```python
from build123d import *

# Parameters (mm, degrees)
F0_W     = 53.4262955189
F0_H     = 38.6142134666
F1_DEPTH = 37.0909944177
F2_R     = 12.7
F3_T     = -2.54


# Not quite as in the source:
# - a shell that OpenCascade refuses in one call is made with other operations: the cavity is built on its own and cut out


with BuildPart() as f1:
    # F0 (on Top) → F1 (new body)
    with BuildSketch(Plane.XY):
        with Locations((-26.7131477594, 19.3071067333)):
            Rectangle(F0_W, F0_H)
    extrude(amount=F1_DEPTH)

    # F2
    f2_edges = [f1.edges().sort_by_distance(p)[0] for p in [
        (-53.426296, 38.614213, 18.545497),
        (-53.426296, 0, 18.545497),
        (-53.426296, 19.307107, 0),
        (-53.426296, 19.307107, 37.090994),
    ]]
    fillet(f2_edges, radius=F2_R)

    # F3: a shell. OpenCascade refuses it in one call, so the cavity is built on its own and cut out:
    # the body offset inwards by the wall thickness, plus a prism from it out through each open face.
    f3_core = offset(f1.part, amount=F3_T, mode=Mode.PRIVATE)
    f3_exits = [f3_core.faces().sort_by_distance(p)[0] for p in [
        (-21.633148, 19.307107, 34.550994),
    ]]
    add(f3_core, mode=Mode.SUBTRACT)
    extrude(f3_exits, amount=-F3_T, mode=Mode.SUBTRACT)


solid = f1.part
```
Input: part model. Units: mm. Frame: model coordinates. A direction names the side the tool comes from. Give positions to 0.01 mm unless a question says otherwise; leave off trailing zeros. Order: outer loops, then holes, each group sorted by start corner. A loop starts at its lowest first (then second) coordinate and runs counter-clockwise, first axis right, second up. Notation, with made-up numbers: M 86.25,77.5 L 122.25,77.5 A28 cw 122.25,112.5 Z; hole C 18,38.25 d8. An arc over 180 degrees is marked long. Return JSON: item names as keys, results as strings.
1) Mould query, pull axis X, two halves, no side actions, for faces 4 (the face through (-48.125, 2.377, 18.805)), 5 (the face through (-21, 20, 0)), 6 (the face through (-46.645, 34.172, 18.77)). Classes: released by +X, released by -X, zero draft, split by the parting line, or undercut.
Taken from the geometry:
{"face 4": "released by -X", "face 5": "zero draft", "face 6": "undercut"}
2) Section query A-A on z = 19. Output: boundary loops of the cut face in (x, y).
Taken from the geometry:
{"outline": "M -53.43,12.7 A12.7 ccw -40.73,0 L 0,0 L 0,38.61 L -40.73,38.61 A12.7 ccw -53.43,25.91 Z; hole M -50.89,12.7 A10.16 ccw -40.73,2.54 L -2.54,2.54 L -2.54,36.07 L -40.73,36.07 A10.16 ccw -50.89,25.91 Z"}
3) Section query D-D on x = -42.5. Output: boundary loops of the cut face in (y, z).
Taken from the geometry:
{"outline": "M 0.12,0.12 L 38.49,0.12 L 38.49,36.97 L 0.12,36.97 Z; hole M 2.7,2.7 L 35.92,2.7 L 35.92,34.39 L 2.7,34.39 Z"}
4) Access query for faces 1 (the face through (-46.64, 19.54, 4.44)), 2 (the face through (-40.726, 19, 36)), 3 (the face through (-2, 17, 37.091)). Directions: +Z, -Z, +X, -X, +Y, -Y. A direction counts if a zero-diameter tool reaches every point of the face in a straight line with its end or side. Return the directions, or none.
Taken from the geometry:
{"face 1": "none", "face 2": "+Z", "face 3": "+Z, +X, -X, +Y, -Y"}
5) Contact query for flat-ended pins moving along their axis: pin 1 (1.5 mm diameter, centred on y = 19.5, z = 10, fed in from -X); pin 2 (5 mm diameter, centred on y = 14, z = 4, fed in from -X). Output: stop coordinate, or through.
Taken from the geometry:
{"pin 1": "stops at x = -53.28", "pin 2": "stops at x = -51.81"}
6) Line query: L1, parallel to X at y = 20.5, z = 22; L2, parallel to Y at x = -34.5, z = 10; L3, parallel to Z at x = -3, y = 10.5. Output: solid intervals per line, ascending. Write a range as [from, to].
Taken from the geometry:
{"L1": "x = [-53.43, -50.89], [-2.54, 0]", "L2": "y = [0, 2.54], [36.07, 38.61]", "L3": "z = [0, 2.54]"}
7) Section query B-B on x = -31. Output: boundary loops of the cut face in (y, z).
Taken from the geometry:
{"outline": "M 0,0 L 38.61,0 L 38.61,37.09 L 36.07,37.09 L 36.07,2.54 L 2.54,2.54 L 2.54,37.09 L 0,37.09 Z"}
8) Section query C-C on y = 21. Output: boundary loops of the cut face in (x, z), and give its area (3 significant figures).
Taken from the geometry:
{"outline": "M -53.43,12.7 A12.7 ccw -40.73,0 L 0,0 L 0,37.09 L -2.54,37.09 L -2.54,2.54 L -40.73,2.54 A10.16 cw -50.89,12.7 L -50.89,24.39 A10.16 cw -40.73,34.55 L -40.73,37.09 A12.7 ccw -53.43,24.39 Z", "area": "312 mm2"}
